from build123d import *

# Parameters (mm, degrees)
BOSS_EXTRUDE1_DEPTH = 430


with BuildPart() as part:
    # Sketch1 → Boss-Extrude1 (new body)
    with BuildSketch(Plane.XY):
        Polygon((-8, 0), (8, 0), (8, 3.35), (6.47, 6), (8, 8.65), (8, 9), (-8, 9), (-8, 8.65), (-6.47, 6), (-8, 3.35), align=None)
    extrude(amount=BOSS_EXTRUDE1_DEPTH)

    # Sketch2 → Cut-Revolve1 (revolve, cut)
    with BuildSketch(Plane.XY.offset(15), mode=Mode.PRIVATE) as cut_revolve1_sk:
        Polygon((0, 9), (4, 9), (4, 3.5), (2.25, 3.5), (2.25, 0), (0, 0), align=None)
    revolve(cut_revolve1_sk.sketch.rotate(Axis((0, 0, 15), (0, 1, 0)), 270), axis=Axis((0, 0, 15), (0, 1, 0)), mode=Mode.SUBTRACT)

    # Sketch3 → Cut-Revolve2 (revolve, cut)
    with BuildSketch(Plane.XY.offset(55), mode=Mode.PRIVATE) as cut_revolve2_sk:
        Polygon((0, 9), (4, 9), (4, 3.5), (2.25, 3.5), (2.25, 0), (0, 0), align=None)
    revolve(cut_revolve2_sk.sketch.rotate(Axis((0, 0, 55), (0, 1, 0)), 270), axis=Axis((0, 0, 55), (0, 1, 0)), mode=Mode.SUBTRACT)

    # Sketch4 → Cut-Revolve3 (revolve, cut)
    with BuildSketch(Plane.XY.offset(95), mode=Mode.PRIVATE) as cut_revolve3_sk:
        Polygon((0, 9), (4, 9), (4, 3.5), (2.25, 3.5), (2.25, 0), (0, 0), align=None)
    revolve(cut_revolve3_sk.sketch.rotate(Axis((0, 0, 95), (0, 1, 0)), 270), axis=Axis((0, 0, 95), (0, 1, 0)), mode=Mode.SUBTRACT)

    # Sketch5 → Cut-Revolve4 (revolve, cut)
    with BuildSketch(Plane.XY.offset(135), mode=Mode.PRIVATE) as cut_revolve4_sk:
        Polygon((0, 9), (4, 9), (4, 3.5), (2.25, 3.5), (2.25, 0), (0, 0), align=None)
    revolve(cut_revolve4_sk.sketch.rotate(Axis((0, 0, 135), (0, 1, 0)), 270), axis=Axis((0, 0, 135), (0, 1, 0)), mode=Mode.SUBTRACT)

    # Sketch6 → Cut-Revolve5 (revolve, cut)
    with BuildSketch(Plane.XY.offset(175), mode=Mode.PRIVATE) as cut_revolve5_sk:
        Polygon((0, 9), (4, 9), (4, 3.5), (2.25, 3.5), (2.25, 0), (0, 0), align=None)
    revolve(cut_revolve5_sk.sketch.rotate(Axis((0, 0, 175), (0, 1, 0)), 270), axis=Axis((0, 0, 175), (0, 1, 0)), mode=Mode.SUBTRACT)

    # Sketch7 → Cut-Revolve6 (revolve, cut)
    with BuildSketch(Plane.XY.offset(215), mode=Mode.PRIVATE) as cut_revolve6_sk:
        Polygon((0, 9), (4, 9), (4, 3.5), (2.25, 3.5), (2.25, 0), (0, 0), align=None)
    revolve(cut_revolve6_sk.sketch.rotate(Axis((0, 0, 215), (0, 1, 0)), 270), axis=Axis((0, 0, 215), (0, 1, 0)), mode=Mode.SUBTRACT)

    # Sketch8 → Cut-Revolve7 (revolve, cut)
    with BuildSketch(Plane.XY.offset(255), mode=Mode.PRIVATE) as cut_revolve7_sk:
        Polygon((0, 9), (4, 9), (4, 3.5), (2.25, 3.5), (2.25, 0), (0, 0), align=None)
    revolve(cut_revolve7_sk.sketch.rotate(Axis((0, 0, 255), (0, 1, 0)), 270), axis=Axis((0, 0, 255), (0, 1, 0)), mode=Mode.SUBTRACT)

    # Sketch9 → Cut-Revolve8 (revolve, cut)
    with BuildSketch(Plane.XY.offset(295), mode=Mode.PRIVATE) as cut_revolve8_sk:
        Polygon((0, 9), (4, 9), (4, 3.5), (2.25, 3.5), (2.25, 0), (0, 0), align=None)
    revolve(cut_revolve8_sk.sketch.rotate(Axis((0, 0, 295), (0, 1, 0)), 270), axis=Axis((0, 0, 295), (0, 1, 0)), mode=Mode.SUBTRACT)

    # Sketch10 → Cut-Revolve9 (revolve, cut)
    with BuildSketch(Plane.XY.offset(335), mode=Mode.PRIVATE) as cut_revolve9_sk:
        Polygon((0, 9), (4, 9), (4, 3.5), (2.25, 3.5), (2.25, 0), (0, 0), align=None)
    revolve(cut_revolve9_sk.sketch.rotate(Axis((0, 0, 335), (0, 1, 0)), 270), axis=Axis((0, 0, 335), (0, 1, 0)), mode=Mode.SUBTRACT)

    # Sketch11 → Cut-Revolve10 (revolve, cut)
    with BuildSketch(Plane.XY.offset(375), mode=Mode.PRIVATE) as cut_revolve10_sk:
        Polygon((0, 9), (4, 9), (4, 3.5), (2.25, 3.5), (2.25, 0), (0, 0), align=None)
    revolve(cut_revolve10_sk.sketch.rotate(Axis((0, 0, 375), (0, 1, 0)), 270), axis=Axis((0, 0, 375), (0, 1, 0)), mode=Mode.SUBTRACT)

    # Sketch12 → Cut-Revolve11 (revolve, cut)
    with BuildSketch(Plane.XY.offset(415), mode=Mode.PRIVATE) as cut_revolve11_sk:
        Polygon((0, 9), (4, 9), (4, 3.5), (2.25, 3.5), (2.25, 0), (0, 0), align=None)
    revolve(cut_revolve11_sk.sketch.rotate(Axis((0, 0, 415), (0, 1, 0)), 270), axis=Axis((0, 0, 415), (0, 1, 0)), mode=Mode.SUBTRACT)


solid = part.part
Check sheet for the modelled part. Datum: model origin and axes. Units: mm. Round coordinates to 2 decimals unless told otherwise and drop trailing zeros. Loops run counter-clockwise (first coordinate to the right, second up) from the corner with the lowest first, then second, coordinate; pieces in that order, holes last.
1. Sectioned sample at A-A on z = 186.5. Record the boundary of the cut face in (x, y), and give its area (3 significant figures).
2. Scan lines: probe 1 along X at (y, z) = (2.4, 295); probe 2 along Y at (x, z) = (7.25, 85); probe 3 along X at (y, z) = (5.8, 95). Record each from-to range of solid material in increasing order.
3. Mould release check, pull along Z, two halves, no side actions. Record for faces 1 (the flat face through (0, 5, 430)), 2 (the flat face through (-2, 3.5, 257)), 3 (the flat face through (0, 5, 0)), 4 (the flat face through (4, 9, 212)): released by +Z, released by -Z, zero draft, split by the parting line, or undercut.
4. Gauge pin test, flat end, axial feed: pin 1 Ø6 at (x, z) = (0, 375) entering from +Y. Record the tip position at first contact, or that the pin passes through.
Recorded:
1. outline: (-8, 0) - (8, 0) - (8, 3.35) - (6.47, 6) - (8, 8.65) - (8, 9) - (-8, 9) - (-8, 8.65) - (-6.47, 6) - (-8, 3.35) - close
1. area: 136 mm2
2. probe 1: x = -8 to -2.25, 2.25 to 8
2. probe 2: y = 0 to 4.65, 7.35 to 9
2. probe 3: x = -6.59 to -4, 4 to 6.59
3. face 1: released by +Z
3. face 2: undercut
3. face 3: released by -Z
3. face 4: zero draft
4. pin 1: stops at y = 3.5
